from build123d import *

# Parameters (mm, degrees)
SKETCH_1_R          = 8.5
EXTRUDE_1_DEPTH     = 2.8
SKETCH_2_R          = 5.955
EXTRUDE_2_DEPTH     = 2.4
SKETCH_3_R          = 7.145
EXTRUDE_3_DEPTH     = 7.4
CHAMFER_1_SIZE      = 0.5
CHAMFER_2_SIZE      = 0.5
CUT_EXTRUDE_1_DEPTH = 5.2
SKETCH_5_R          = 3.464101615
CUT_EXTRUDE_2_DEPTH = 0.5
CUT_EXTRUDE_2_DRAFT = -37


with BuildPart() as part:
    # 草图1 → 拉伸1 (new body)
    with BuildSketch(Plane.XY):
        Circle(SKETCH_1_R)
    extrude(amount=EXTRUDE_1_DEPTH)

    # 草图2 → 拉伸2 (add)
    with BuildSketch(Plane.XY.offset(2.8)):
        Circle(SKETCH_2_R)
    extrude(amount=EXTRUDE_2_DEPTH)

    # 草图3 → 拉伸3 (add)
    with BuildSketch(Plane.XY.offset(5.2)):
        Circle(SKETCH_3_R)
    extrude(amount=EXTRUDE_3_DEPTH)

    # 倒角1
    chamfer_1_edges = [part.edges().sort_by_distance(p)[0] for p in [
        (-7.145, 0, 12.6),
    ]]
    chamfer(chamfer_1_edges, length=CHAMFER_1_SIZE)

    # 倒角2
    chamfer_2_edges = [part.edges().sort_by_distance(p)[0] for p in [
        (-8.5, 0, 0),
    ]]
    chamfer(chamfer_2_edges, length=CHAMFER_2_SIZE)

    # 草图4 → 切除-拉伸1 (cut)
    with BuildSketch(Plane(origin=(0, 0, 0), x_dir=(-1, 0, 0), z_dir=(0, 0, -1))):
        Polygon((2.258087232, -2.626983451), (3.40407802, 0.642069181), (1.145990788, 3.269052632), (-2.258087232, 2.626983451), (-3.40407802, -0.642069181), (-1.145990788, -3.269052632), align=None)
    extrude(amount=-CUT_EXTRUDE_1_DEPTH, mode=Mode.SUBTRACT)


with BuildPart() as cut_extrude_2_tool:
    # 草图5 → 切除-拉伸2 (with draft: the straight prism first)
    with BuildSketch(Plane(origin=(0, 0, 0), x_dir=(-1, 0, 0), z_dir=(0, 0, -1))):
        Circle(SKETCH_5_R)
    extrude(amount=-CUT_EXTRUDE_2_DEPTH)
    # 切除-拉伸2: the draft: its side faces are tilted about the plane it starts from
    cut_extrude_2_sides = [cut_extrude_2_tool.faces().sort_by_distance(p)[0] for p in [
        (3.464101615, 0, 0.25),
    ]]
    draft(cut_extrude_2_sides, Plane(origin=(0, 0, 0), x_dir=(-1, 0, 0), z_dir=(0, 0, -1)), CUT_EXTRUDE_2_DRAFT)


with BuildPart() as part_1:
    add(part.part)

    # 切除-拉伸2: cut by cut_extrude_2_tool
    add(cut_extrude_2_tool.part, mode=Mode.SUBTRACT)


solid = part_1.part
Geometry: final body of the model. Coordinates: model frame, mm. A direction names the side the tool comes from. Coordinates: 2 decimals unless noted, no trailing zeros. Order: outer loops, then holes, each group sorted by start corner. A loop starts at its lowest first (then second) coordinate and runs counter-clockwise, first axis right, second up.
(1) Section query A-A (z = 3.5). Return the cut outline in (x, y) (3 decimals).
(2) Access query for faces 5 (the face through (0, 0, 12.6)), 6 (the face through (-4.73, -3.62, 3.98)), 7 (the face through (-2.82, -1.02, 2.56)). Directions: +Z, -Z, +X, -X, +Y, -Y. A direction counts if a zero-diameter tool reaches every point of the face in a straight line with its end or side. Return the directions, or none.
(3) Draft query along X for faces 1 (the face through (-2.5, 2.12, 0.25)), 2 (the face through (3.297, -6.339, 8.602)), 3 (the face through (-2, 6, 5.2)), 4 (the face through (3.086, 1.107, 0.247)). Return one class per face: pulls with the +X half, pulls with the -X half, needs draft (parallel to the pull), parting line crosses it, or undercut.
(4) Section query C-C (y = 0). Return the cut outline in (x, z) (3 decimals), plus the area to 3 significant figures.
(5) Section query D-D (z = 1.5). Return the cut outline in (x, y), plus the area to 3 significant figures.
(6) Material intervals for probe 1 along Z at (x, y) = (-0.25, 1); probe 2 along Z at (x, y) = (-7.5, 0.5); probe 3 along X at (y, z) = (2.5, 1.75), sorted ascending.
(7) Section query B-B (z = 10.25). Return the cut outline in (x, y) (3 decimals).
(8) First-contact query: pin 1 (5 mm diameter, centred on y = 2, z = 7, fed in from -X) (3 decimals); pin 2 (6 mm diameter, centred on x = 6, z = 8, fed in from -Y); pin 3 (1 mm diameter, centred on x = -2, y = 2, fed in from -Z). Flat tips, straight axial feed; report the tip coordinate or a pass-through.
Solution:
1. outline: circle Ø11.91 at (0, 0); hole (-3.404, 0.642) - (-2.258, -2.627) - (1.146, -3.269) - (3.404, -0.642) - (2.258, 2.627) - (-1.146, 3.269) - close
2. face 5: +Z, +X, -X, +Y, -Y
2. face 6: none
2. face 7: -Z
3. face 1: undercut
3. face 2: parting line crosses it
3. face 3: needs draft
3. face 4: undercut
4. outline: (-8.5, 0.5) - (-8, 0) - (-3.464, 0) - (-3.179, 0.378) - (-3.179, 5.2) - (3.179, 5.2) - (3.179, 0.378) - (3.464, 0) - (8, 0) - (8.5, 0.5) - (8.5, 2.8) - (5.955, 2.8) - (5.955, 5.2) - (7.145, 5.2) - (7.145, 12.1) - (6.645, 12.6) - (-6.645, 12.6) - (-7.145, 12.1) - (-7.145, 5.2) - (-5.955, 5.2) - (-5.955, 2.8) - (-8.5, 2.8) - close
4. area: 148 mm2
5. outline: circle Ø17 at (0, 0); hole (-3.4, 0.64) - (-2.26, -2.63) - (1.15, -3.27) - (3.4, -0.64) - (2.26, 2.63) - (-1.15, 3.27) - close
5. area: 196 mm2
6. probe 1: z = 5.2 to 12.6
6. probe 2: z = 0 to 2.8
6. probe 3: x = -8.12 to -1.81, 2.3 to 8.12
7. outline: circle Ø14.29 at (0, 0)
8. pin 1: stops at x = -7.145
8. pin 2: stops at y = -6.48
8. pin 3: stops at z = 0.18
